Part print with two shaded views. Sizes in mm from the minimum x, y, z corner. A direction names the side the tool comes from. Round coordinates to 2 decimals unless told otherwise and drop trailing zeros. Order: outer loops, then holes, each group sorted by start corner. A loop starts at its lowest first (then second) coordinate and runs counter-clockwise, first axis right, second up. Notation, with made-up numbers: (-29.5, -34) - (28.5, -34) arc R26 ccw to (28.5, 3) - close; hole circle Ø3 at (75.25, 61). An arc over 180 degrees is marked (long way). Write item = value, one per line.
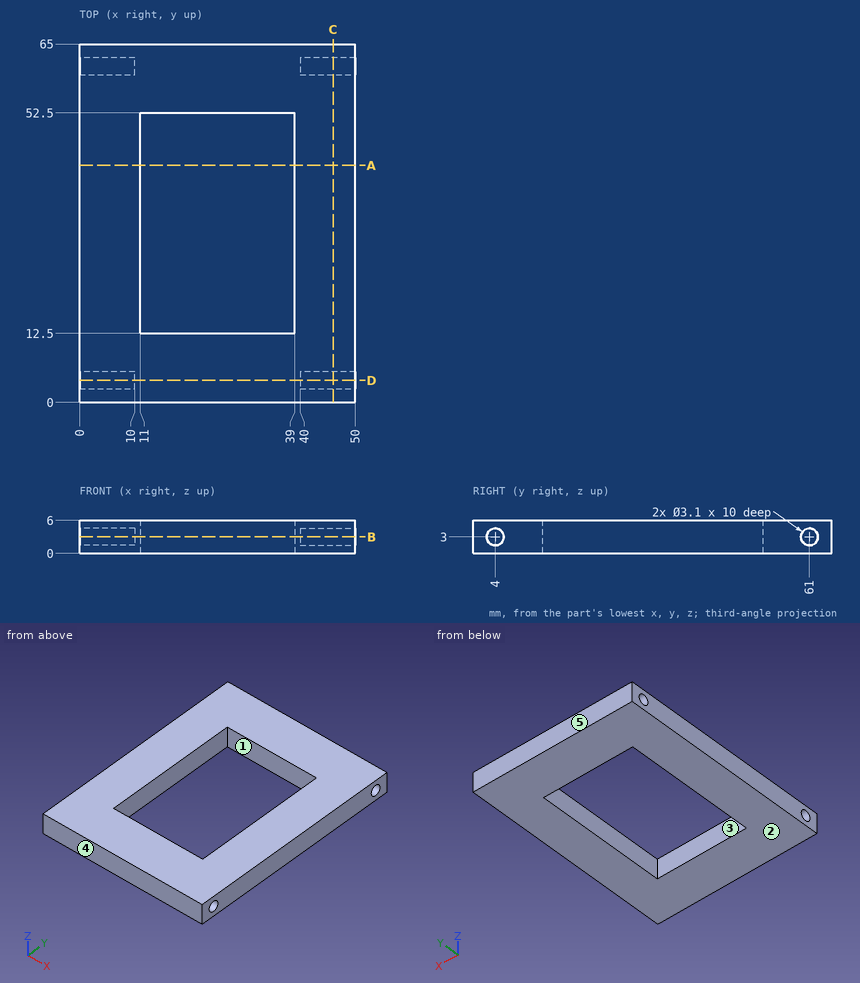
1) Cut at C-C (x = 46). Write the cut outline in (y, z), and give its area (3 significant figures).
Conclusion:
outline = (0, 0) - (65, 0) - (65, 6) - (0, 6) - close; hole circle Ø3.1 at (4, 3); hole circle Ø3.1 at (61, 3)
area = 375 mm^2
2) Cut at B-B (z = 3). Write the cut outline in (x, y).
Conclusion:
outline = (0, 0) - (50, 0) - (50, 2.45) - (40, 2.45) - (40, 5.55) - (50, 5.55) - (50, 59.45) - (40, 59.45) - (40, 62.55) - (50, 62.55) - (50, 65) - (0, 65) - (0, 62.55) - (10, 62.55) - (10, 59.45) - (0, 59.45) - (0, 5.55) - (10, 5.55) - (10, 2.45) - (0, 2.45) - close; hole (11, 12.5) - (39, 12.5) - (39, 52.5) - (11, 52.5) - close
3) Mould opens along Y. For the marked faces 3, 4 and 5 say: +Y half, -Y half, draft (parallel to the pull), parting line (faces both ways), or undercut.
Conclusion:
face_3 = undercut
face_4 = -Y half
face_5 = +Y half
4) Wall check: line 1 along X through (y, z) = (47, 4.1); line 2 along Z through (x, y) = (3.75, 4); line 3 along Y through (x, z) = (29, 4.9). Give the ranges that are in metal, low to high.
Conclusion:
line_1 = 0 to 11, 39 to 50
line_2 = 0 to 1.45, 4.55 to 6
line_3 = 0 to 12.5, 52.5 to 65
5) 3-axis set-ups, long thin cutter, end or side, ignore diameter. For the marked faces 1 and 2: which of +Z, -Z, +X, -X, +Y, -Y reach the whole face in a straight line?
Conclusion:
face_1 = +Z, -Z
face_2 = -Z, +X, -X, +Y, -Y
6) Cut at D-D (y = 4). Write the cut outline in (x, z).
Conclusion:
outline = (0, 0) - (50, 0) - (50, 1.45) - (40, 1.45) - (40, 4.55) - (50, 4.55) - (50, 6) - (0, 6) - (0, 4.55) - (10, 4.55) - (10, 1.45) - (0, 1.45) - close
7) Cut at A-A (y = 43). Write the cut outline in (x, z).
Conclusion:
outline = (0, 0) - (11, 0) - (11, 6) - (0, 6) - close; (39, 0) - (50, 0) - (50, 6) - (39, 6) - close
8) Flat gauge pin, fed straight in: pin 1 Ø1.5 at (y, z) = (4, 3) entering from +X. Where does the tip first touch, or does it go through?
Conclusion:
pin_1 = 40
